Source: three-view drawing plus pictorial views. Frame: mm from the lowest corner of the part. Give positions to 0.01 mm unless a question says otherwise; leave off trailing zeros. Order: outer loops, then holes, each group sorted by start corner. A loop starts at its lowest first (then second) coordinate and runs counter-clockwise, first axis right, second up. Notation, with made-up numbers: M 69.25,-0.5 L 120.25,-0.5 A26 cw 120.25,36.5 Z; hole C 13.25,35 d10. An arc over 180 degrees is marked long. Use CSV: the item, a comma, the result in double quotes.
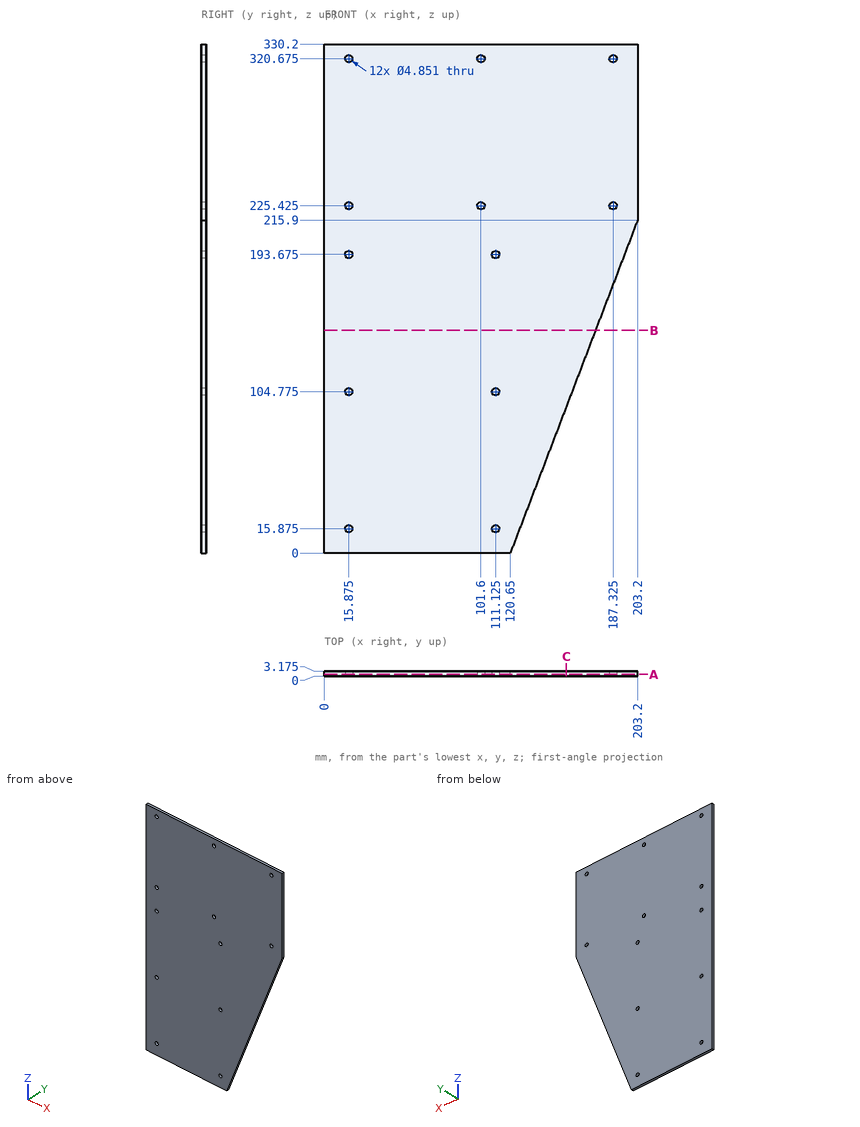
1. Section B-B, the plane z = 144.5. Return the cut outline in (x, y) (1 decimal).
Answer:
outline,"M 0,0 L 175.9,0 L 175.9,3.2 L 0,3.2 Z"
2. Section C-C, the plane x = 157. Return the cut outline in (y, z) (1 decimal).
Answer:
outline,"M 0,95.1 L 3.2,95.1 L 3.2,330.2 L 0,330.2 Z"
3. Section A-A, the plane y = 1.05. Give the number of separate pieces and of enclosed holes in the cut face, plus the area to 3 significant figures.
Answer:
separate pieces,"1"
enclosed holes,"12"
area,"58,000 mm2"
4. Line query: line 1 (X direction, y = 1.15, z = 199); line 2 (X direction, y = 2.05, z = 117.5). Output: solid intervals per line, ascending.
Answer:
line 1,"0 to 196.74"
line 2,"0 to 165.58"
5. Pin query (flat end, axial travel): pin 1 Ø3 at (x, z) = (15.875, 193.675) entering from -Y. Return the tip coordinate at first contact, or that it passes through.
Answer:
pin 1,"through"
